from build123d import *

# Parameters (mm, degrees)
BOSS_EXTRU_1_DEPTH = 5
FILLET1_R          = 2


with BuildPart() as part:
    # Esquisse1 → Boss.-Extru.1 (new body)
    with BuildSketch(Plane.XY):
        Polygon((1.7, 70), (1.7, 65), (0, 65), (0, 25), (-2, 25), (-2, 20), (0, 20), (0, 16.5), (2, 16.5), (2, 17.6), (4.3, 17.6), (4.3, 16.5), (7, 16.5), (7, 13.5), (4.3, 13.5), (4.3, 12.4), (2, 12.4), (2, 13.5), (0, 13.5), (0, 10), (-2, 10), (-2, 5), (0, 5), (0, 0), (23.4, 0), (23.4, 5), (25.4, 5), (25.4, 10), (23.4, 10), (23.4, 13.5), (21.4, 13.5), (21.4, 12.4), (19.1, 12.4), (19.1, 13.5), (16.4, 13.5), (16.4, 16.5), (19.1, 16.5), (19.1, 17.6), (21.4, 17.6), (21.4, 16.5), (23.4, 16.5), (23.4, 20), (25.4, 20), (25.4, 25), (23.4, 25), (23.4, 65), (21.7, 65), (21.7, 70), (16.7, 70), (16.7, 65), (13.2, 65), (13.2, 62), (14.3, 62), (14.3, 59.7), (13.2, 59.7), (13.2, 55), (10.2, 55), (10.2, 59.7), (9.1, 59.7), (9.1, 62), (10.2, 62), (10.2, 65), (6.7, 65), (6.7, 70), align=None)
    extrude(amount=BOSS_EXTRU_1_DEPTH)

    # Fillet1
    fillet1_edges = [part.edges().sort_by_distance(p)[0] for p in [
        (23.4, 0, 2.5),
        (0, 0, 2.5),
    ]]
    fillet(fillet1_edges, radius=FILLET1_R)


solid = part.part
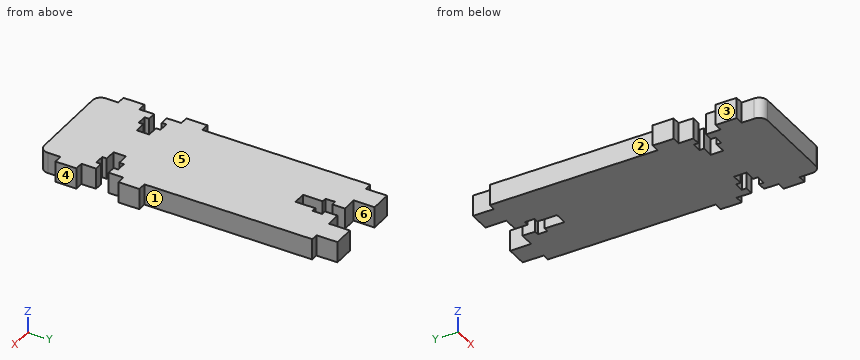
CAD build for the part. Positions are in the model's coordinates, mm. Face numbers are marked on the shaded views. A direction names the side the tool comes from. Give positions to 0.01 mm unless a question says otherwise; leave off trailing zeros. Write each loop counter-clockwise with the first axis right and the second up, starting at its lowest first coordinate (ties: lowest second). Pieces come first, ordered by that corner, then holes. Notation, with made-up numbers: (46, 34.25) - (85, 34.25) arc R22 cw to (85, 63.25) - close; hole circle Ø9 at (67.25, 44.5). An arc over 180 degrees is marked (long way). Put each result on its own line as item: value.
(1) Pull direction X, two halves, no side cores. Call the marked faces 4, 5 and 6: released by +X, released by -X, zero draft, split by the parting line, or undercut.
Working result:
face 4: released by +X
face 5: zero draft
face 6: undercut
(2) Saw through at A-A (x = 2.75). List the corners of the cut face in (y, z), then the cut area to 3 significant figures.
Working result:
outline: (0, 0) - (12.4, 0) - (12.4, 5) - (0, 5) - close; (17.6, 0) - (70, 0) - (70, 5) - (17.6, 5) - close
area: 324 mm^2
(3) Saw through at D-D (x = 12). List the corners of the cut face in (y, z).
Working result:
outline: (0, 0) - (55, 0) - (55, 5) - (0, 5) - close
(4) Saw through at C-C (y = 32). List the corners of the cut face in (x, z), then the cut area to 3 significant figures.
Working result:
outline: (0, 0) - (23.4, 0) - (23.4, 5) - (0, 5) - close
area: 117 mm^2
(5) Wall check: L1, parallel to Y at x = 5, z = 2.6; L2, parallel to Y at x = 2.25, z = 4.55; L3, parallel to X at y = 4, z = 2.25. Give the ranges that are in metal, low to high.
Working result:
L1: 0 to 13.5, 16.5 to 70
L2: 0 to 12.4, 17.6 to 70
L3: 0 to 23.4
(6) Saw through at B-B (y = 64). List the corners of the cut face in (x, z), then the cut area to 3 significant figures.
Working result:
outline: (0, 0) - (10.2, 0) - (10.2, 5) - (0, 5) - close; (13.2, 0) - (23.4, 0) - (23.4, 5) - (13.2, 5) - close
area: 102 mm^2
(7) Drop flat-ended pins along their axis: pin 1 Ø0.5 at (y, z) = (12.5, 2.5) entering from -X; pin 2 Ø3 at (y, z) = (12.5, 3) entering from +X; pin 3 Ø0.8 at (x, z) = (22, 2) entering from +Y; pin 4 Ø1 at (x, z) = (0.5, 3.5) entering from -Y. Give the stop position or say it passes through.
Working result:
pin 1: x = 0
pin 2: x = 23.4
pin 3: y = 70
pin 4: y = 0.27
(8) Tool access for the marked faces 1, 2 and 3: list every direction of +Z, -Z, +X, -X, +Y, -Y with a clear straight run to the whole face (end or side of a thin tool).
Working result:
face 1: +Z, -Z, +X, +Y
face 2: +Z, -Z, -X, +Y
face 3: +Z, -Z, -X, +Y, -Y
